For this review, take the finished solid that the model builds, in its own axes (mm). Face numbers are marked on the shaded views. A direction names the side the tool comes from. Coordinates: 2 decimals unless noted, no trailing zeros. Order: outer loops, then holes, each group sorted by start corner. A loop starts at its lowest first (then second) coordinate and runs counter-clockwise, first axis right, second up. Notation, with made-up numbers: M 51,-9 L 85,-9 A33 cw 85,26 Z; hole C 80.25,-31 d9. An arc over 180 degrees is marked long. Use CSV: the item, a comma, the result in double quotes.
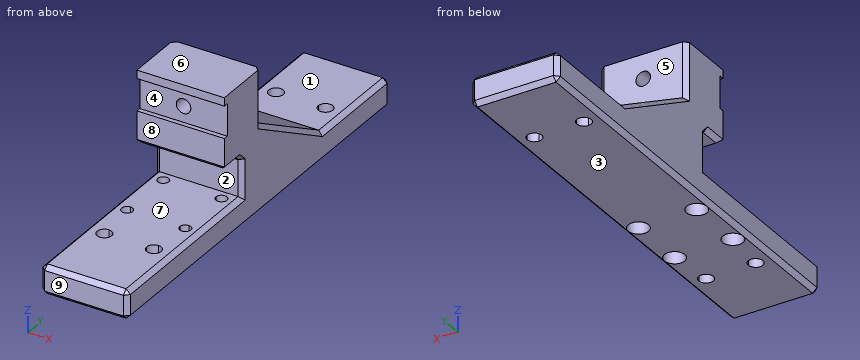
```python
from build123d import *

# Parameters (mm, degrees)
SKETCH1_W           = 30
SKETCH1_H           = 145
BOSS_EXTRUDE1_DEPTH = 10
CUT_EXTRUDE1_DEPTH  = 32
CUT_EXTRUDE2_DEPTH  = 32
SKETCH4_R           = 3.5
CUT_EXTRUDE3_DEPTH  = 5
SKETCH5_W           = 30
SKETCH5_H           = 10
BOSS_EXTRUDE2_DEPTH = 39
SKETCH6_W           = 30
SKETCH6_H           = 25
BOSS_EXTRUDE3_DEPTH = 10
SKETCH7_W           = 11
SKETCH7_H           = 1.6
CUT_EXTRUDE4_DEPTH  = 61
SKETCH8_R           = 2.5
CUT_EXTRUDE5_DEPTH  = 61
CHAMFER1_SIZE       = 20
CHAMFER1_SIZE2      = 34.641016151
CHAMFER2_SIZE       = 1.5


with BuildPart() as part:
    # Sketch1 → Boss-Extrude1 (new body)
    with BuildSketch(Plane.XY):
        with Locations((15, 72.5)):
            Rectangle(SKETCH1_W, SKETCH1_H)
    extrude(amount=BOSS_EXTRUDE1_DEPTH)

    # Sketch2 → Cut-Extrude1 (cut)
    with BuildSketch(Plane.XY.offset(10)):
        with BuildLine():
            Line((6.5, 117.5), (6.5, 120))
            Line((6.5, 120), (9, 120))
            ThreePointArc((9, 120), (4.732233047, 121.767766953), (6.5, 117.5))
        make_face()
        with BuildLine():
            Line((9, 120), (6.5, 120))
            Line((6.5, 120), (6.5, 117.5))
            ThreePointArc((6.5, 117.5), (8.267766953, 118.232233047), (9, 120))
        make_face()
        with BuildLine():
            ThreePointArc((26, 120), (23.5, 122.5), (21, 120))
            Line((21, 120), (23.5, 120))
            Line((23.5, 120), (23.5, 117.5))
            ThreePointArc((23.5, 117.5), (25.267766953, 118.232233047), (26, 120))
        make_face()
        with BuildLine():
            Line((23.5, 120), (21, 120))
            ThreePointArc((21, 120), (21.732233047, 118.232233047), (23.5, 117.5))
            Line((23.5, 117.5), (23.5, 120))
        make_face()
        with BuildLine():
            ThreePointArc((26, 25), (25.267766953, 26.767766953), (23.5, 27.5))
            Line((23.5, 27.5), (23.5, 25))
            Line((23.5, 25), (21, 25))
            ThreePointArc((21, 25), (23.5, 22.5), (26, 25))
        make_face()
        with BuildLine():
            Line((23.5, 25), (23.5, 27.5))
            ThreePointArc((23.5, 27.5), (21.732233047, 26.767766953), (21, 25))
            Line((21, 25), (23.5, 25))
        make_face()
        with BuildLine():
            ThreePointArc((9, 25), (8.267766953, 26.767766953), (6.5, 27.5))
            Line((6.5, 27.5), (6.5, 25))
            Line((6.5, 25), (9, 25))
        make_face()
        with BuildLine():
            Line((6.5, 25), (6.5, 27.5))
            ThreePointArc((6.5, 27.5), (4.732233047, 23.232233047), (9, 25))
            Line((9, 25), (6.5, 25))
        make_face()
    extrude(amount=-CUT_EXTRUDE1_DEPTH, mode=Mode.SUBTRACT)

    # Sketch3 → Cut-Extrude2 (cut)
    with BuildSketch(Plane.XY.offset(10)):
        with BuildLine():
            ThreePointArc((6.9, 60), (3.656497116, 61.343502884), (5, 58.1))
            Line((5, 58.1), (5, 60))
            Line((5, 60), (6.9, 60))
        make_face()
        with BuildLine():
            Line((5, 60), (5, 58.1))
            ThreePointArc((5, 58.1), (6.343502884, 58.656497116), (6.9, 60))
            Line((6.9, 60), (5, 60))
        make_face()
        with BuildLine():
            ThreePointArc((23.1, 60), (23.656497116, 58.656497116), (25, 58.1))
            Line((25, 58.1), (25, 60))
            Line((25, 60), (23.1, 60))
        make_face()
        with BuildLine():
            Line((25, 60), (25, 58.1))
            ThreePointArc((25, 58.1), (26.343502884, 58.656497116), (26.9, 60))
            ThreePointArc((26.9, 60), (25, 61.9), (23.1, 60))
            Line((23.1, 60), (25, 60))
        make_face()
        with BuildLine():
            Line((5, 41.9), (5, 40))
            Line((5, 40), (6.9, 40))
            ThreePointArc((6.9, 40), (6.343502884, 41.343502884), (5, 41.9))
        make_face()
        with BuildLine():
            Line((6.9, 40), (5, 40))
            Line((5, 40), (5, 41.9))
            ThreePointArc((5, 41.9), (3.656497116, 38.656497116), (6.9, 40))
        make_face()
        with BuildLine():
            ThreePointArc((25, 41.9), (23.656497116, 41.343502884), (23.1, 40))
            Line((23.1, 40), (25, 40))
            Line((25, 40), (25, 41.9))
        make_face()
        with BuildLine():
            Line((25, 40), (23.1, 40))
            ThreePointArc((23.1, 40), (25, 38.1), (26.9, 40))
            ThreePointArc((26.9, 40), (26.343502884, 41.343502884), (25, 41.9))
            Line((25, 41.9), (25, 40))
        make_face()
    extrude(amount=-CUT_EXTRUDE2_DEPTH, mode=Mode.SUBTRACT)

    # Sketch4 → Cut-Extrude3 (cut)
    with BuildSketch(Plane(origin=(0, 0, 0), x_dir=(-1, 0, 0), z_dir=(0, 0, -1))):
        with Locations((-5, 60)):
            Circle(SKETCH4_R)
        with Locations((-5, 40)):
            Circle(SKETCH4_R)
        with Locations((-25, 40)):
            Circle(SKETCH4_R)
        with Locations((-25, 60)):
            Circle(SKETCH4_R)
    extrude(amount=-CUT_EXTRUDE3_DEPTH, mode=Mode.SUBTRACT)

    # Sketch5 → Boss-Extrude2 (add)
    with BuildSketch(Plane.XY.offset(10)):
        with Locations((15, 68.5)):
            Rectangle(SKETCH5_W, SKETCH5_H)
    extrude(amount=BOSS_EXTRUDE2_DEPTH)

    # Sketch6 → Boss-Extrude3 (add)
    with BuildSketch(Plane.XZ.offset(-63.5)):
        with Locations((15, 36.5)):
            Rectangle(SKETCH6_W, SKETCH6_H)
    extrude(amount=BOSS_EXTRUDE3_DEPTH)

    # Sketch7 → Cut-Extrude4 (cut)
    with BuildSketch(Plane(origin=(30, 0, 0), x_dir=(0, 0, -1), z_dir=(1, 0, 0))):
        with Locations((-40.675105606, 54.3)):
            Rectangle(SKETCH7_W, SKETCH7_H)
    extrude(amount=-CUT_EXTRUDE4_DEPTH, mode=Mode.SUBTRACT)

    # Sketch8 → Cut-Extrude5 (cut)
    with BuildSketch(Plane.XZ.offset(-55.1)):
        with Locations(Location((15, 40.675105606, 0), (0, 0, 270))):
            Circle(SKETCH8_R)
    extrude(amount=-CUT_EXTRUDE5_DEPTH, mode=Mode.SUBTRACT)

    # Chamfer1
    chamfer1_edges = [part.edges().sort_by_distance(p)[0] for p in [
        (15, 73.5, 10),
    ]]
    chamfer1_side = [part.faces().sort_by_distance(p)[0] for p in [
        (15, 73.5, 29.309258212),
    ]]
    chamfer(chamfer1_edges, length=CHAMFER1_SIZE, length2=CHAMFER1_SIZE2, reference=chamfer1_side[0])

    # Chamfer2
    chamfer2_edges = [part.edges().sort_by_distance(p)[0] for p in [
        (30, 63.5, 17),
        (0, 63.5, 17),
        (15, 63.5, 24),
        (0, 58.5, 24),
        (30, 58.5, 24),
        (15, 53.5, 24),
        (30, 31.75, 10),
        (30, 126.570508076, 10),
        (0, 90.820508076, 20),
        (30, 90.820508076, 20),
        (15, 145, 10),
        (0, 126.570508076, 10),
        (15, 145, 0),
        (30, 72.5, 0),
        (15, 0, 0),
        (0, 72.5, 0),
        (0, 145, 5),
        (30, 145, 5),
        (30, 0, 5),
        (0, 0, 5),
        (15, 0, 10),
        (0, 31.75, 10),
        (0, 73.5, 39.5),
        (30, 73.5, 39.5),
    ]]
    chamfer(chamfer2_edges, length=CHAMFER2_SIZE - 0.0001)  # a hair under: the kernel refuses the full size


solid = part.part
```
Item 1: Clearance check with flat-ended pins moving along their axes: pin 1 Ø4.5 at (x, y) = (5, 40) entering from +Z; pin 2 Ø1 at (x, y) = (10, 90) entering from +Z; pin 3 Ø14 at (x, z) = (11, 16) entering from -Y. State where each tip first meets the part, or that it passes through.
Solutions:
pin 1,"z = 10"
pin 2,"z = 20.76"
pin 3,"y = 0.5"
Item 2: To check wall thickness, follow line 1 along Y through (x, z) = (5, 7); line 2 along Y through (x, z) = (18.5, 40.5); line 3 along Z through (x, y) = (8, 52.5). State the ranges of each line that lie inside material, in increasing order. Write a range as [from, to].
Solutions:
line 1,"[0, 23], [27, 38.1], [41.9, 58.1], [61.9, 118], [122, 145]"
line 2,"[55.1, 73.5]"
line 3,"[0, 10]"
Item 3: Draft analysis for pull direction Z (two halves, no side actions). For the marked faces 1, 2, 3 and 4, state which applies: released by +Z, released by -Z, zero draft, split by the parting line, or undercut.
Solutions:
face 1,"released by +Z"
face 2,"undercut"
face 3,"released by -Z"
face 4,"undercut"
Item 4: Add section B-B on z = 21. State the section outline as (x, y) points, and give its area (3 significant figures).
Solutions:
outline,"M 0,65 L 1.5,63.5 L 28.5,63.5 L 30,65 L 30,86.09 L 28.5,89.09 L 1.5,89.09 L 0,86.09 Z"
area,"761 mm^2"
Item 5: For the marked faces 5, 6, 7, 8 and 9, list the 3-axis set-ups (+Z, -Z, +X, -X, +Y, -Y) from which the entire face can be reached by the end or side of a thin tool; tool diameter is ignored.
Solutions:
face 5,"+Z, +X, -X, +Y"
face 6,"+Z, +X, -X, +Y, -Y"
face 7,"+X, -X, -Y"
face 8,"+Z, +X, -X, -Y"
face 9,"+Z, -Z, +X, -X, -Y"
Item 6: Add section C-C on x = 10.5. State the section outline as (y, z) points, and give its area (3 significant figures).
Solutions:
outline,"M 0,1.5 L 1.5,0 L 143.5,0 L 145,1.5 L 145,8.5 L 143.5,10 L 108.14,10 L 73.5,30 L 73.5,49 L 53.5,49 L 53.5,46.18 L 55.1,46.18 L 55.1,35.18 L 53.5,35.18 L 53.5,25.5 L 55,24 L 62,24 L 63.5,22.5 L 63.5,10 L 1.5,10 L 0,8.5 Z"
area,"2,410 mm^2"
Item 7: Add section A-A on y = 111. State the section outline as (x, z) points, and give its area (4 significant figures).
Solutions:
outline,"M 0,1.5 L 1.5,0 L 28.5,0 L 30,1.5 L 30,8.5 L 28.5,10 L 1.5,10 L 0,8.5 Z"
area,"295.5 mm^2"
